Check sheet for the modelled part. Datum: model origin and axes. Units: mm. A direction names the side the tool comes from. Give positions to 0.01 mm unless a question says otherwise; leave off trailing zeros. Loops run counter-clockwise (first coordinate to the right, second up) from the corner with the lowest first, then second, coordinate; pieces in that order, holes last. Notation, with made-up numbers: (14, 23.5) - (72, 23.5) arc R14 cw to (72, 40.5) - close; hole circle Ø6 at (15, 28). An arc over 180 degrees is marked (long way). Use one line per item in the form item = value.
from build123d import *

# Parameters (mm, degrees)
F1_DEPTH  = 127
F2_R      = 5.08
F3_W      = 88.9
F3_H      = 55.88
F4_DEPTH  = 12.7
F5_R      = 5.08
F6_W      = 196.3208343999
F6_H      = 25.4
F7_DEPTH  = 12.7
F8_R      = 5.08
F9_R      = 8.0743885719
F10_DEPTH = 5.08


# Not quite as in the source:
# - a fillet or chamfer that OpenCascade refuses, or shapes differently, is made with other operations: its cross-section is extruded or revolved along the edge and cut away or added


with BuildPart() as f1:
    # F0 (on Right) → F1 (new body, symmetric)
    with BuildSketch(Plane.YZ):
        Polygon((102.2654771805, 0), (102.2654771805, 24.730855599), (-76.7904296517, 0), align=None)
    extrude(amount=F1_DEPTH, both=True)

    # F2
    f2_edges = [f1.edges().sort_by_distance(p)[0] for p in [
        (-127, 12.737524, 12.365428),
        (127, 12.737524, 12.365428),
        (0, 102.265477, 24.730856),
    ]]
    fillet(f2_edges, radius=F2_R)

    # F3 (on face) → F4 (join)
    with BuildSketch(Plane(origin=(0, -1.4374781315, 10.4076039488), x_dir=(1, 0, 0), z_dir=(0, -0.1368192087, 0.9905960348))):
        with Locations((-53.7104171999, 25.7286139321)):
            Rectangle(F3_W, F3_H)
        with Locations((53.7104171999, 25.7286139321)):
            Rectangle(F3_W, F3_H)
        with Locations((53.7104171999, -42.8513860679)):
            Rectangle(F3_W, F3_H)
        with Locations((-53.7104171999, -42.8513860679)):
            Rectangle(F3_W, F3_H)
    extrude(amount=F4_DEPTH)

    # F5
    f5_edges = [f1.edges().sort_by_distance(p)[0] for p in [
        (-98.160417, 22.311581, 26.508342),
        (-53.710417, -5.365672, 22.685613),
        (-98.160417, -45.623495, 17.125281),
        (-53.710417, -73.300748, 13.302552),
        (-53.710417, -17.946242, 20.94801),
        (-9.260417, -45.623495, 17.125281),
        (53.710417, -5.365672, 22.685613),
        (9.260417, 22.311581, 26.508342),
        (53.710417, 49.988834, 30.331071),
        (98.160417, 22.311581, 26.508342),
        (53.710417, -17.946242, 20.94801),
        (9.260417, -45.623495, 17.125281),
        (53.710417, -73.300748, 13.302552),
        (98.160417, -45.623495, 17.125281),
        (-9.260417, 22.311581, 26.508342),
        (-53.710417, 49.988834, 30.331071),
    ]]
    fillet(f5_edges, radius=F5_R)

    # F6 (on face) → F7 (join)
    with BuildSketch(Plane(origin=(0, -1.4374781315, 10.4076039488), x_dir=(1, 0, 0), z_dir=(0, -0.1368192087, 0.9905960348))):
        with Locations((0, 78.1313713312)):
            Rectangle(F6_W, F6_H)
    extrude(amount=F7_DEPTH)

    # F8
    f8_edges = [f1.edges().sort_by_distance(p)[0] for p in [
        (0, 61.640975, 31.940442),
        (0, 86.802114, 35.41565),
        (98.160417, 74.221545, 33.678046),
        (-98.160417, 74.221545, 33.678046),
    ]]
    fillet(f8_edges, radius=F8_R)

    # F9 (on face) → F10 (join)
    with BuildSketch(Plane(origin=(0, 0, 0), x_dir=(1, 0, 0), z_dir=(0, 0, -1))):
        with Locations((-114.6246567369, -91.883122921)):
            Circle(F9_R)
        with Locations((114.6246567369, -91.883122921)):
            Circle(F9_R)
    extrude(amount=F10_DEPTH)

    # F11: fillet of radius 7.62 on 2 edges, made by hand

    # F11_s1 → F11_t2 (revolve, cut)
    with BuildSketch(Plane.XZ.offset(-91.883122921)):
        with BuildLine():
            ThreePointArc((122.6990453088, 0), (119.9142494631, -3.6817039467), (115.5148404119, -5.08))
            Line((115.5148404119, -5.08), (122.6990453088, -5.08))
            Line((122.6990453088, -5.08), (122.6990453088, 0))
        make_face()
    revolve(axis=Axis((114.6246567369, 91.883122921, -5.08), (0, 0, -1)), mode=Mode.SUBTRACT)

    # F11_s3 → F11_t4 (revolve, cut)
    with BuildSketch(Plane.XZ.offset(-91.883122921)):
        with BuildLine():
            ThreePointArc((-106.5502681649, 0), (-109.3350640106, -3.6817039467), (-113.7344730618, -5.08))
            Line((-113.7344730618, -5.08), (-106.5502681649, -5.08))
            Line((-106.5502681649, -5.08), (-106.5502681649, 0))
        make_face()
    revolve(axis=Axis((-114.6246567369, 91.883122921, -5.08), (0, 0, -1)), mode=Mode.SUBTRACT)


solid = f1.part
Item 1: Mould release check, pull along Y, two halves, no side actions. Record for faces 1 (the face through (54.333, -71.657, 11.988)), 2 (the face through (1.374, 63.285, 30.625)), 3 (the face through (2, 102.265, 9)): released by +Y, released by -Y, zero draft, split by the parting line, or undercut.
Answer block:
face_1 = released by -Y
face_2 = undercut
face_3 = released by +Y
Item 2: Gauge pin test, flat ends, axial feed: P1, Ø12, axis at y = 74, z = 23.5, coming from the -X side; P2, Ø1, axis at y = 5, z = 15, coming from the +X side; P3, Ø10, axis at y = -7, z = 28, coming from the +X side; P4, Ø4.5, axis at y = -39.5, z = 10, coming from the -X side. Record the tip position at first contact, or that the pin passes through.
Answer block:
P1 = -126.7
P2 = 98.16
P3 = through
P4 = -98.16
Item 3: Section check A-A on x = 2.5. Record the boundary of the cut face in (y, z).
Answer block:
outline = (-76.79, 0) - (102.27, 0) - (102.27, 18.9) arc R5.08 ccw to (96.49, 23.93) - (88.54, 22.84) - (87.5, 30.38) arc R5.08 ccw to (81.77, 34.72) - (66.67, 32.64) arc R5.08 ccw to (62.34, 26.91) - (63.38, 19.36) - close
Item 4: Thickness scan on L1, parallel to X at y = 50.5, z = 23; L2, parallel to Z at x = 54, y = 46.5; L3, parallel to X at y = 1, z = 19. Record the ranges inside material, lowest first.
Answer block:
L1 = -98.16 to -9.26, 9.26 to 98.16
L2 = 0 to 29.61
L3 = -98.13 to -9.29, 9.29 to 98.13
Item 5: Access from +Z, -Z, +X, -X, +Y, -Y to the whole of each face (thin tool, end or side, straight path). Record for faces 4 (the face through (53.088, 51.212, 21.472)), 5 (the face through (98.16, -45, 8)), 6 (the face through (-98.16, -45, 8)).
Answer block:
face_4 = +Z, +X, -X
face_5 = +Z, +X, -Y
face_6 = +Z, -X, -Y
